```python
from build123d import *

# Parameters (mm, degrees)
F1_DEPTH = 66.04
F2_R     = 33.01999
F4_W     = 9.652
F4_H     = 28.448
F5_DEPTH = 30.226
F3_R     = 11.1125
F6_DEPTH = 63.246


# Not quite as in the source:
# - a fillet or chamfer is up to 0.001 mm smaller than in the source, because OpenCascade refuses the exact size


with BuildPart() as f1:
    # F0 (on Front) → F1 (new body)
    with BuildSketch(Plane.XZ):
        Polygon((0, 19.304), (0, 0), (38.608, 0), (38.608, 86.36), (19.304, 86.36), (19.304, 19.304), align=None)
    extrude(amount=F1_DEPTH)

    # F2 (radius 33.02 in the source; OpenCascade refuses exactly that, so slightly less here)
    f2_edges = [f1.edges().sort_by_distance(p)[0] for p in [
        (28.956, -66.04, 86.36),
        (28.956, 0, 86.36),
    ]]
    fillet(f2_edges, radius=F2_R)

    # F4 (on face) → F5 (cut)
    with BuildSketch(Plane.XY.offset(19.304)):
        with Locations((4.826, -33.02)):
            Rectangle(F4_W, F4_H)
    extrude(amount=-F5_DEPTH, mode=Mode.SUBTRACT)

    # F3 (on face) → F6 (cut)
    with BuildSketch(Plane(origin=(19.304, 0, 0), x_dir=(0, -1, 0), z_dir=(-1, 0, 0))):
        with Locations((33.02, 53.34)):
            Circle(F3_R)
    extrude(amount=-F6_DEPTH, mode=Mode.SUBTRACT)


solid = f1.part
```
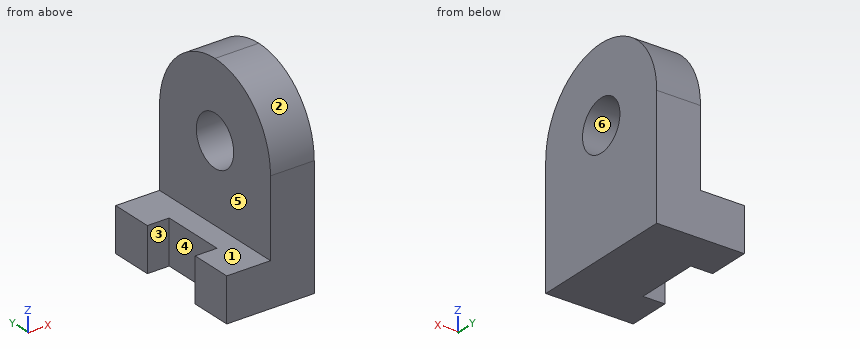
Design review of the part built by this model. Coordinates are the model's own, in mm. Face numbers are marked on the shaded views. A direction names the side the tool comes from. Round coordinates to 2 decimals unless told otherwise and drop trailing zeros. Order: outer loops, then holes, each group sorted by start corner. A loop starts at its lowest first (then second) coordinate and runs counter-clockwise, first axis right, second up. Notation, with made-up numbers: M 43.25,80.25 L 70.25,80.25 A25 cw 70.25,102.25 Z; hole C -26.75,71.25 d4. An arc over 180 degrees is marked long. Put each result on its own line as item: value.
Q1. Consider section D-D (x = 16). State the section outline as (y, z) points, and give its area (3 significant figures).
Reported:
outline: M -66.04,0 L 0,0 L 0,19.3 L -66.04,19.3 Z
area: 1,270 mm²
Q2. Draft analysis for pull direction Y (two halves, no side actions). For the marked faces 1, 2 and 3, state which applies: released by +Y, released by -Y, zero draft, split by the parting line, or undercut.
Reported:
face 1: zero draft
face 2: released by -Y
face 3: undercut
Q3. Consider section A-A (z = 60). State the section outline as (x, y) points.
Reported:
outline: M 19.3,-65.36 L 38.61,-65.36 L 38.61,-41.92 L 19.3,-41.92 Z; M 19.3,-24.12 L 38.61,-24.12 L 38.61,-0.68 L 19.3,-0.68 Z
Q4. To check wall thickness, follow line 1 (Y direction, x = 23.5, z = 53); line 2 (Z direction, x = 32, y = -33); line 3 (X direction, y = -57, z = 60.5). State the ranges of each line that lie inside material, in increasing order.
Reported:
line 1: -66.04 to -44.13, -21.91 to 0
line 2: 0 to 42.23, 64.45 to 86.36
line 3: 19.3 to 38.61
Q5. Machinability: for the marked faces 4, 5 and 6, which of the approach directions +Z, -Z, +X, -X, +Y, -Y give a long, thin tool a straight path to every point of the face, cutting with its end or side? Answer none if there is none.
Reported:
face 4: +Z, -Z, -X
face 5: +Z, -X, +Y, -Y
face 6: +X, -X
Q6. Insertion check: pin 1 Ø7.5 at (x, z) = (6.5, 8) entering from +Y; pin 2 Ø2 at (x, z) = (30, 77) entering from -Y; pin 3 Ø6 at (y, z) = (-30, 13.5) entering from -X; pin 4 Ø1 at (x, y) = (8.5, -42) entering from -Z. Each pin has a flat end and moves straight along its axis. Give the tip position at first contact, or say it passes through.
Reported:
pin 1: y = 0
pin 2: y = -57.04
pin 3: x = 9.65
pin 4: through
Q7. Consider section C-C (z = 30). State the section outline as (x, y) points, and give its area (3 significant figures).
Reported:
outline: M 19.3,-66.04 L 38.61,-66.04 L 38.61,0 L 19.3,0 Z
area: 1,270 mm²
